from build123d import *

# Parameters (mm, degrees)
F0_W     = 76.2
F0_H     = 76.2
F0_R     = 4
F1_DEPTH = 2.6416
F2_R     = 5.08
F3_W     = 40.450208
F3_H     = 43.757458
F4_DEPTH = 37.592
F5_R     = 5.08
F7_DEPTH = 16.256


with BuildPart() as f1:
    # F0 (on Top) → F1 (new body)
    with BuildSketch(Plane.XY):
        Rectangle(F0_W, F0_H)
        with Locations((-28.1, -28.1)):
            Circle(F0_R, mode=Mode.SUBTRACT)
        with Locations((28.1, -28.1)):
            Circle(F0_R, mode=Mode.SUBTRACT)
        with Locations((-28.1, 28.1)):
            Circle(F0_R, mode=Mode.SUBTRACT)
        with Locations((28.1, 28.1)):
            Circle(F0_R, mode=Mode.SUBTRACT)
    extrude(amount=F1_DEPTH)

    # F2
    f2_edges = [f1.edges().sort_by_distance(p)[0] for p in [
        (-38.1, -38.1, 1.3208),
        (38.1, -38.1, 1.3208),
        (38.1, 38.1, 1.3208),
        (-38.1, 38.1, 1.3208),
    ]]
    fillet(f2_edges, radius=F2_R)

    # F3 (on face) → F4 (join)
    with BuildSketch(Plane.XY.offset(2.6416)):
        Rectangle(F3_W, F3_H)
    extrude(amount=F4_DEPTH)

    # F5
    f5_edges = [f1.edges().sort_by_distance(p)[0] for p in [
        (-20.225104, -21.878729, 21.4376),
        (20.225104, -21.878729, 21.4376),
        (20.225104, 21.878729, 21.4376),
        (-20.225104, 21.878729, 21.4376),
    ]]
    fillet(f5_edges, radius=F5_R)

    # F6 (on face) → F7 (cut)
    with BuildSketch(Plane.XY.offset(40.2336)):
        with BuildLine():
            Line((-16.923103, 16.798729), (-16.923103, -16.798729))
            ThreePointArc((-16.923103, -16.798729), (-16.402339, -18.055964), (-15.145104, -18.576728))
            Line((-15.145104, -18.576728), (15.145104, -18.576728))
            ThreePointArc((15.145104, -18.576728), (16.402339, -18.055964), (16.923103, -16.798729))
            Line((16.923103, -16.798729), (16.923103, 16.798729))
            ThreePointArc((16.923103, 16.798729), (16.402339, 18.055964), (15.145104, 18.576728))
            Line((15.145104, 18.576728), (-15.145104, 18.576728))
            ThreePointArc((-15.145104, 18.576728), (-16.402339, 18.055964), (-16.923103, 16.798729))
        make_face()
    extrude(amount=-F7_DEPTH, mode=Mode.SUBTRACT)


solid = f1.part
Can you work these out from the model? Positions are in its coordinate system, mm. A direction names the side the tool comes from. Coordinates: 2 decimals unless noted, no trailing zeros. Order: outer loops, then holes, each group sorted by start corner. A loop starts at its lowest first (then second) coordinate and runs counter-clockwise, first axis right, second up. Notation, with made-up numbers: M 18.25,59.25 L 34.25,59.25 A13 ccw 34.25,69.25 Z; hole C -31,69.25 d1. An arc over 180 degrees is marked long. Answer as CSV lines item,"result".
(1) Suppose I cut it at D-D on y = -15. Please give me the cut outline in (x, z).
Geometry check:
outline,"M -38.1,0 L 38.1,0 L 38.1,2.64 L 20.23,2.64 L 20.23,40.23 L 16.92,40.23 L 16.92,23.98 L -16.92,23.98 L -16.92,40.23 L -20.23,40.23 L -20.23,2.64 L -38.1,2.64 Z"
(2) I'm going to push flat-ended pins straight in: pin 1 (12 mm diameter, centred on x = -8.5, y = 0, fed in from +Z); pin 2 (10.5 mm diameter, centred on x = -28.1, y = -28.1, fed in from -Z); pin 3 (9 mm diameter, centred on x = 28.1, y = 28.1, fed in from +Z); pin 4 (4 mm diameter, centred on x = 17, z = 18.5, fed in from +Y). Where does each tip first touch, or does it pass through?
Geometry check:
pin 1,"z = 23.98"
pin 2,"z = 0"
pin 3,"z = 2.64"
pin 4,"y = 21.88"
(3) Please list where these lines run through material, in increasing order: L1, parallel to Y at x = 28.1, z = 0.75; L2, parallel to X at y = 10.5, z = 25.
Geometry check:
L1,"-38.1 to -32.1, -24.1 to 24.1, 32.1 to 38.1"
L2,"-20.23 to -16.92, 16.92 to 20.23"
(4) Suppose I cut it at A-A on y = -28.1. Please give me the cut outline in (x, z).
Geometry check:
outline,"M -38.1,0 L -32.1,0 L -32.1,2.64 L -38.1,2.64 Z; M -24.1,0 L 24.1,0 L 24.1,2.64 L -24.1,2.64 Z; M 32.1,0 L 38.1,0 L 38.1,2.64 L 32.1,2.64 Z"
(5) Suppose I cut it at B-B on z = 7.5. Please give me the cut outline in (x, y), plus the area to 3 significant figures.
Geometry check:
outline,"M -20.23,-16.8 A5.08 ccw -15.15,-21.88 L 15.15,-21.88 A5.08 ccw 20.23,-16.8 L 20.23,16.8 A5.08 ccw 15.15,21.88 L -15.15,21.88 A5.08 ccw -20.23,16.8 Z"
area,"1,750 mm^2"
(6) On a 3-axis mill with a long thin cutter (end or side, diameter ignored), from which of +Z, -Z, +X, -X, +Y, -Y can I reach the whole of each face in a straight line? I mean faces 1 (the flat face through (-20.225, 0, 21)), 2 (the cylindrical face through (16.39, -18.07, 32.22)), 3 (the cylindrical face through (18.7, -20.43, 21.7)), 4 (the flat face through (0, -21.879, 21)). Say none if no direction works.
Geometry check:
face 1,"+Z, -X, +Y, -Y"
face 2,"+Z"
face 3,"+Z, +X, -Y"
face 4,"+Z, +X, -X, -Y"
(7) If we mould it in two halves opening along Y, with no side actions, what happens to faces 5 (the flat face through (38.1, 0, 1)), 6 (the cylindrical face through (-16.39, 18.07, 32.22)), 7 (the cylindrical face through (-28.621, -24.134, 1.302)), 8 (the cylindrical face through (36.572, -36.651, 1.339))? For each: released by +Y, released by -Y, zero draft, split by the parting line, or undercut.
Geometry check:
face 5,"zero draft"
face 6,"undercut"
face 7,"undercut"
face 8,"released by -Y"
